from build123d import *

# Parameters (mm, degrees)
EXTRUDE_1_DEPTH          = 6
EXTRUDE_1_DEPTH_BACK     = 6
SKETCH_1_R               = 1.5
SKETCH_1_R_2             = 0.75
CUT_EXTRUDE_1_DEPTH      = 36.391559728
CUT_EXTRUDE_1_DEPTH_BACK = 36.391559728
SKETCH_2_W               = 62.866350052
SKETCH_2_H               = 37.677296861


with BuildPart() as part:
    # Sketch 1 → Extrude 1 (new, two sides: drawn at the far end of the back side and taken through both)
    with BuildSketch(Plane(origin=(0, 0, 0), x_dir=(1, 0, 0), z_dir=(0, 1, 0)).offset(-EXTRUDE_1_DEPTH_BACK)):
        with BuildLine():
            Line((0, 2), (-31.75, 3))
            ThreePointArc((-31.75, 3), (-34.75, 0), (-31.75, -3))
            Line((-31.75, -3), (0, -2))
            ThreePointArc((0, -2), (2, 0), (0, 2))
        make_face()
        with Locations(Location((-31.75, 0, 0), (0, 0, 270))):
            Circle(SKETCH_1_R, mode=Mode.SUBTRACT)
        with Locations(Location((0, 0, 0), (0, 0, 270))):
            Circle(SKETCH_1_R_2, mode=Mode.SUBTRACT)
    extrude(amount=EXTRUDE_1_DEPTH + EXTRUDE_1_DEPTH_BACK)

    # Sketch 2 → Cut-Extrude 1 (cut, two sides: drawn at the far end of the back side and taken through both)
    with BuildSketch(Plane.XY.offset(-CUT_EXTRUDE_1_DEPTH_BACK)):
        with Locations((-15.620530839, 1.877248647)):
            Rectangle(SKETCH_2_W, SKETCH_2_H)
        Polygon((2, 6), (-6.448133576, 6), (-12.448133575, 3), (-28.75, -0.25), (-34.75, -0.25), (-34.75, -2.25), (-28.75, -2.25), (-9.588391111, 1.570128768), (-6.448133576, 0), (2, 0), (2, 2), (-5.975997621, 2), (-7.975997621, 3), (-5.975997621, 4), (2, 4), align=None, mode=Mode.SUBTRACT)
    extrude(amount=CUT_EXTRUDE_1_DEPTH + CUT_EXTRUDE_1_DEPTH_BACK, mode=Mode.SUBTRACT)


solid = part.part
The listing builds one solid part. Answer for the finished solid, in the listing's coordinates (mm). A direction names the side the tool comes from. Give positions to 0.01 mm unless a question says otherwise; leave off trailing zeros. Write each loop counter-clockwise with the first axis right and the second up, starting at its lowest first coordinate (ties: lowest second). Pieces come first, ordered by that corner, then holes.
Item 1: Section B-B, the plane y = -1 is taken. Write down the section's boundary in (x, z), plus the area to 3 significant figures.
Item 2: Which of the six approach directions +Z, -Z, +X, -X, +Y, -Y give full straight-line access (tool end or side, diameter ignored) to faces 1 (the flat face through (-2, 4, 0)), 2 (the flat face through (-2, 0, 0)), 3 (the flat face through (-8.04, 0.796, -0.032)), 4 (the flat face through (-30, -2.25, 0)), 5 (the flat face through (-30, -0.25, -1))?
Item 3: Determine the mould class of faces 6 (the flat face through (-20.48, 1.4, -0.04)), 7 (the cylindrical face through (-30.485, -1.264, 0.806)), 8 (the cylindrical face through (-34.75, -1.26, -0.07)) for opening direction Z: released by +Z, released by -Z, zero draft, split by the parting line, or undercut.
Item 4: Flat-ended cylindrical pins translate along their axes: P1, Ø2.5, axis at x = 0, z = 0, coming from the -Y side; P2, Ø1.5, axis at x = -14.5, z = -0.5, coming from the -Y side; P3, Ø1.8, axis at x = -30.5, z = 0, coming from the +Y side. Find the tip coordinate at first contact, or state that the pin passes through.
Item 5: Find the intervals of material crossed by line 1 along Y through (x, z) = (-1.5, -0.05); line 2 along Z through (x, y) = (-31.75, -1.5); line 3 along Y through (x, z) = (-29, -1.9), in increasing order.
Item 6: Section D-D, the plane x = -23.5 is taken. Write down the section's boundary in (y, z).
Item 7: Section A-A, the plane z = 0 is taken. Write down the section's boundary in (x, y).
Item 8: Section C-C, the plane y = 2.5 is taken. Write down the section's boundary in (x, z).
Completed:
1. outline: (-31.75, -3) - (-22.48, -2.71) - (-22.48, 2.71) - (-31.75, 3) arc R3 ccw to start; hole circle Ø3 at (-31.75, 0)
1. area: 60.0 mm2
2. face 1: +Z, -Z, +X
2. face 2: +Z, -Z, +X, -Y
2. face 3: +Z, -Z, -Y
2. face 4: +Z, -Z, +X, -X, -Y
2. face 5: +Z, -Z, -X, +Y
3. face 6: zero draft
3. face 7: undercut
3. face 8: split by the parting line
4. P1: stops at y = 0
4. P2: stops at y = 0.44
4. P3: stops at y = -0.25
5. line 1: y = 0 to 2, 4 to 6
5. line 2: z = -3 to -1.5, 1.5 to 3
5. line 3: y = -2.25 to -0.25
6. outline: (-1.2, -2.74) - (0.8, -2.74) - (0.8, 2.74) - (-1.2, 2.74) - close
7. outline: (-34.75, -2.25) - (-33.25, -2.25) - (-33.25, -0.25) - (-34.75, -0.25) - close; (-30.25, -2.25) - (-28.75, -2.25) - (-9.59, 1.57) - (-6.45, 0) - (-0.75, 0) - (-0.75, 2) - (-5.98, 2) - (-7.98, 3) - (-5.98, 4) - (-0.75, 4) - (-0.75, 6) - (-6.45, 6) - (-12.45, 3) - (-28.75, -0.25) - (-30.25, -0.25) - close; (0.75, 0) - (2, 0) - (2, 2) - (0.75, 2) - close; (0.75, 4) - (2, 4) - (2, 6) - (0.75, 6) - close
8. outline: (-14.96, -2.47) - (-6.98, -2.22) - (-6.98, 2.22) - (-14.96, 2.47) - close
